Verification items for this drawing (mm, ordinates from the low corner). Round coordinates to 2 decimals unless told otherwise and drop trailing zeros. Write each loop counter-clockwise with the first axis right and the second up, starting at its lowest first coordinate (ties: lowest second). Pieces come first, ordered by that corner, then holes.
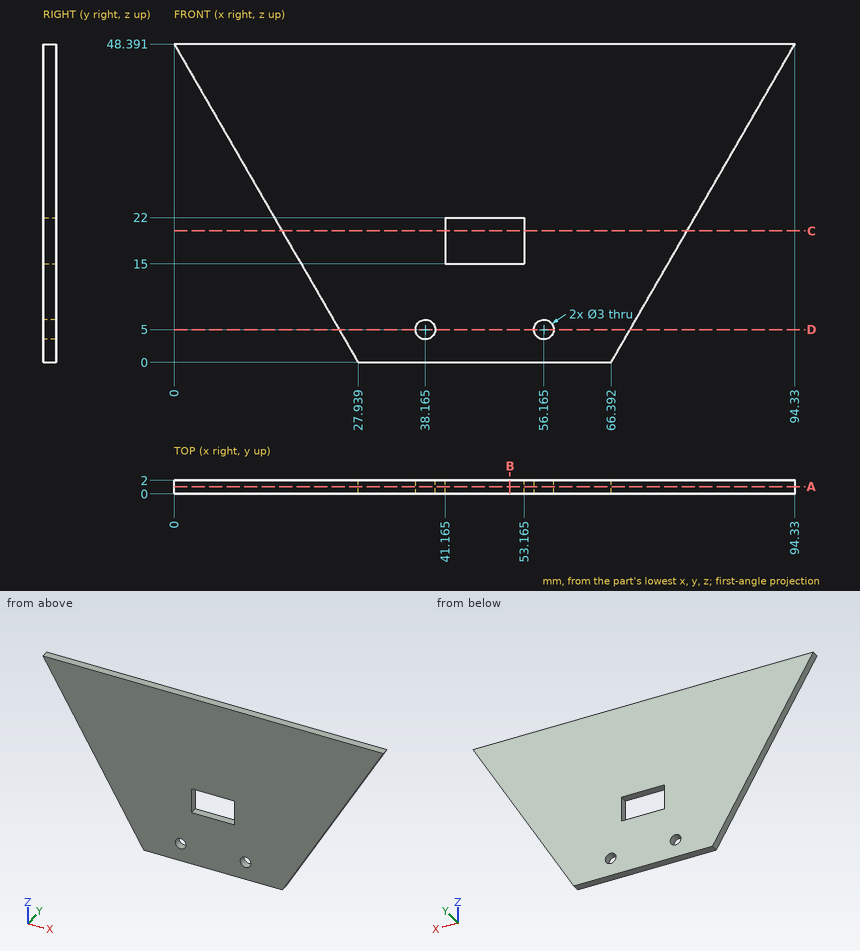
1. Section check A-A (y = 1.05). Record the cut outline in (x, z) (1 decimal).
2. Section check C-C (z = 20). Record the cut outline in (x, y) (1 decimal).
3. Section check B-B (x = 51). Record the cut outline in (y, z).
4. Scan lines: line 1 along Z through (x, y) = (41.5, 0.25); line 2 along Z through (x, y) = (55, 0.8) (1 decimal); line 3 along X through (y, z) = (0.8, 4) (1 decimal). Record each from-to range of solid material in increasing order.
5. Depth check by flat-ended pin: pin 1 Ø0.6 at (x, y) = (47, 1) entering from -Z; pin 2 Ø1.8 at (x, z) = (56.17, 5) entering from +Y; pin 3 Ø1 at (y, z) = (1, 17) entering from -X (1 decimal). Enter the tip coordinate at first touch or a pass-through.
6. Section check D-D (z = 5). Record the cut outline in (x, y) (1 decimal).
Results below:
1. outline: (0, 48.4) - (27.9, 0) - (66.4, 0) - (94.3, 48.4) - close; hole circle Ø3 at (38.2, 5); hole (41.2, 15) - (53.2, 15) - (53.2, 22) - (41.2, 22) - close; hole circle Ø3 at (56.2, 5)
2. outline: (16.4, 0) - (41.2, 0) - (41.2, 2) - (16.4, 2) - close; (53.2, 0) - (77.9, 0) - (77.9, 2) - (53.2, 2) - close
3. outline: (0, 0) - (2, 0) - (2, 15) - (0, 15) - close; (0, 22) - (2, 22) - (2, 48.39) - (0, 48.39) - close
4. line 1: z = 0 to 15, 22 to 48.39
4. line 2: z = 0 to 4.1, 5.9 to 48.4
4. line 3: x = 25.6 to 37, 39.3 to 55, 57.3 to 68.7
5. pin 1: stops at z = 0
5. pin 2: passes through
5. pin 3: stops at x = 17.8
6. outline: (25.1, 0) - (36.7, 0) - (36.7, 2) - (25.1, 2) - close; (39.7, 0) - (54.7, 0) - (54.7, 2) - (39.7, 2) - close; (57.7, 0) - (69.3, 0) - (69.3, 2) - (57.7, 2) - close
